Read the model definition and answer for the solid it produces. Units are mm, in the model's axes. A direction names the side the tool comes from. Round coordinates to 2 decimals unless told otherwise and drop trailing zeros. Write each loop counter-clockwise with the first axis right and the second up, starting at its lowest first coordinate (ties: lowest second). Pieces come first, ordered by that corner, then holes. Notation, with made-up numbers: (50, -39) - (86, -39) arc R34 ccw to (86, -8) - close; hole circle Ø5 at (17, 74.25). An arc over 180 degrees is marked (long way). One line per item, written item: value. Start each with the question number.
(1) The mould has two halves that part along X. Classify faces 4 (the face through (12.932, -0.493, 5.362)), 5 (the face through (5.1, -1, 9.4)), 6 (the face through (-23.75, 1.52, -0.08)): +X half, -X half, draft (parallel to the pull), parting line (faces both ways), or undercut.
(2) A cutting plane is placed at A-A, the plane z = 0. State how many separate pieces and enclosed holes the cut face has, plus the area to 3 significant figures.
(3) A cutting plane is placed at C-C, the plane y = -8.25. Determine the outline of the cut face in (x, z), plus the area to 3 significant figures.
(4) Flat-ended cylindrical pins translate along their axes: pin 1 Ø4 at (x, z) = (-15.56, -15.56) entering from +Y; pin 2 Ø8 at (x, z) = (0, 0) entering from -Y; pin 3 Ø12 at (x, z) = (-8.5, 13) entering from -Y; pin 4 Ø2 at (x, z) = (15.56, -15.56) entering from +Y. Find the tip coordinate at first contact, or state that the pin passes through.
(5) For faces 1 (the face through (-12, 0, -12)), 2 (the face through (-13.887, 1.521, 15.031)), 3 (the face through (-12, 3, -12)), determine the directions among +Z, -Z, +X, -X, +Y, -Y from which every point of the face is accessible in a straight line to the end or side of a thin tool.
(6) A cutting plane is placed at D-D, the plane z = -22. Determine the outline of the cut face in (x, y).
(7) A cutting plane is placed at B-B, the plane x = -22. Determine the outline of the cut face in (y, z), plus the area to 3 significant figures.
(8) Find the intervals of material crossed by L1, parallel to Z at x = 0, y = -8; L2, parallel to Y at x = -4, z = 0.5; L3, parallel to Z at x = 6, y = -4, in increasing order.
Autodesk Inventor part; units mm, degrees
ref_plane "YZ Plane" through (0, 0, 0) normal (1, 0, 0) x (0, 1, 0)
ref_plane "XZ Plane" through (0, 0, 0) normal (0, 1, 0) x (-1, 0, 0)
ref_plane "XY Plane" through (0, 0, 0) normal (0, 0, 1) x (1, 0, 0)
sketch "Sketch1" plane through (0, 0, 0) normal (0, 1, 0) x (-1, 0, 0)
  circle A0 centre (0, 0) radius 27
  dimension "d0" = 54
extrude "Extrusion1" add sketch "Sketch1" along normal blind 3
sketch "Sketch2" plane through (0, 3, 0) normal (0, 1, 0) x (1, 0, 0)
  circle A0 centre (0, 0) radius 16
  dimension "d3" = 32
extrude "Extrusion2" add sketch "Sketch2" along normal blind 1.5
sketch "Sketch3" plane through (0, 0, 0) normal (0, -1, 0) x (1, 0, 0)
  circle A0 centre (0, 0) radius 14
  dimension "d6" = 28
extrude "Extrusion3" add sketch "Sketch3" along normal blind 1
sketch "Sketch4" plane through (0, 4.5, 0) normal (0, 1, 0) x (1, 0, 0)
  circle A0 centre (0, 0) radius 3
  dimension "d9" = 6
extrude "Extrusion4" cut sketch "Sketch4" against normal through all
sketch "Sketch5" plane through (0, -1, 0) normal (0, -1, 0) x (1, 0, 0)
  circle A0 centre (0, 0) radius 6.5
  circle A1 centre (0, 0) radius 10.5
  dimension "d12" = 13
  dimension "d16" = 21
extrude "Extrusion6" add sketch "Sketch5" along normal blind 9.5
fillet "Fillet1" radius 2 1 edges at (-6.5, -1, 0)
sketch "Sketch7" plane through (0, 3, 0) normal (0, 1, 0) x (1, 0, 0)
  circle A0 centre (0, 0) radius 3 construction
  circle A1 centre (0, 0) radius 22 construction
  circle A2 centre (-22, 0) radius 1.75
  circle A3 centre (-15.5563, -15.5563) radius 1.75
  circle A4 centre (0, -22) radius 1.75
  circle A5 centre (15.5563, -15.5563) radius 1.75
  circle A6 centre (22, 0) radius 1.75
  circle A7 centre (15.5563, 15.5563) radius 1.75
  circle A8 centre (0, 22) radius 1.75
  circle A9 centre (-15.5563, 15.5563) radius 1.75
  dimension "d20" = 44
  dimension "d22" = 3.5
  dimension "d25" = 360
extrude "Extrusion7" cut sketch "Sketch7" against normal through all
properties part number "reverse gear lower cylinder cover"
Here are the results:
1. face 4: parting line
1. face 5: draft
1. face 6: undercut
2. separate pieces: 4
2. enclosed holes: 0
2. area: 262 mm²
3. outline: circle Ø21 at (0, 0); hole circle Ø13 at (0, 0)
3. area: 214 mm²
4. pin 1: y = 3
4. pin 2: y = -1
4. pin 3: y = -10.5
4. pin 4: through
5. face 1: -Y
5. face 2: +Y, -Y
5. face 3: +Y
6. outline: (-15.65, 0) - (-1.75, 0) - (-1.75, 3) - (-15.65, 3) - close; (1.75, 0) - (15.65, 0) - (15.65, 3) - (1.75, 3) - close
7. outline: (0, -15.65) - (3, -15.65) - (3, -1.75) - (0, -1.75) - close; (0, 1.75) - (3, 1.75) - (3, 15.65) - (0, 15.65) - close
7. area: 83.4 mm²
8. L1: -10.5 to -6.5, 6.5 to 10.5
8. L2: -1 to 4.5
8. L3: -8.62 to -2.5, 2.5 to 8.62
